Autodesk Inventor part; units mm, degrees
ref_plane "YZ Plane" through (0, 0, 0) normal (1, 0, 0) x (0, 1, 0)
ref_plane "XZ Plane" through (0, 0, 0) normal (0, 1, 0) x (-1, 0, 0)
ref_plane "XY Plane" through (0, 0, 0) normal (0, 0, 1) x (1, 0, 0)
sketch "Boceto1" plane through (0, 0, 0) normal (0, 1, 0) x (-1, 0, 0)
  line L0 (-5, 0) -> (-75.1, 0)
  line L1 (-80.1, -5) -> (-80.1, -91.5)
  line L2 (-75.1, -96.5) -> (-5, -96.5)
  line L3 (0, -91.5) -> (0, -5)
  arc A0 (0, -5) -> (-5, 0) centre (-5, -5) ccw
  arc A1 (-75.1, 0) -> (-80.1, -5) centre (-75.1, -5) ccw
  arc A2 (-80.1, -91.5) -> (-75.1, -96.5) centre (-75.1, -91.5) ccw
  arc A3 (-5, -96.5) -> (0, -91.5) centre (-5, -91.5) ccw
  point P0 (0, 0)
  point P1 (-80.1, -96.5)
  point P2 (-80.1, 0)
  point P3 (0, -96.5)
  dimension "d0" = 96.5
  dimension "d1" = 80.1
  dimension "d2" = 5
extrude "Extrusión1" add sketch "Boceto1" along normal blind 6
sketch "Boceto2" plane through (0, 0, 0) normal (0, -1, 0) x (1, 0, 0)
  circle A0 centre (10.2, -10.54) radius 2.5
  circle A1 centre (10.2, -16.54) radius 2.5
  circle A2 centre (7.06, -57.64) radius 2.4
  circle A3 centre (7.06, -62.64) radius 2.4
  circle A4 centre (7.06, -67.64) radius 2.4
  circle A5 centre (7.08, -75.21) radius 2.4
  circle A6 centre (7.08, -80.21) radius 2.4
  circle A7 centre (7.08, -85.21) radius 2.4
  point P0 (0, 0)
extrude "Extrusión2" cut sketch "Boceto2" against normal blind 10
sketch "Boceto3" plane through (0, 6, 0) normal (0, 1, 0) x (1, 0, 0)
  line L0 (6.9461, 7.6948) -> (13.2683, 7.6948)
  line L1 (13.2683, 7.6948) -> (13.2683, 19.5905)
  line L2 (13.2683, 19.5905) -> (6.9461, 19.5905)
  line L3 (6.9461, 19.5905) -> (6.9461, 7.6948)
  circle A0 centre (10.2, 16.54) radius 2.5
  circle A1 centre (10.2, 10.54) radius 2.5
  point P0 (0, 0)
extrude "Extrusión3" add sketch "Boceto3" along normal blind 15
fillet "Empalme1" radius 3 4 edges at (6.9461, 13.5, -19.5905) (6.9461, 13.5, -7.6948) (13.2683, 13.5, -7.6948) (13.2683, 13.5, -19.5905)
sketch "Boceto4" plane through (0, 6, 0) normal (0, 1, 0) x (1, 0, 0)
  line L0 (3.9852, 54.3304) -> (10.0586, 54.3304)
  line L1 (10.0586, 54.3304) -> (10.0586, 88.8384)
  line L2 (10.0586, 88.8384) -> (3.9852, 88.8384)
  line L3 (3.9852, 88.8384) -> (3.9852, 54.3304)
  circle A0 centre (7.06, 57.64) radius 2.4
  circle A1 centre (7.06, 62.64) radius 2.4
  circle A2 centre (7.06, 67.64) radius 2.4
  circle A3 centre (7.08, 75.21) radius 2.4
  circle A4 centre (7.08, 80.21) radius 2.4
  circle A5 centre (7.08, 85.21) radius 2.4
  point P0 (0, 0)
extrude "Extrusión4" add sketch "Boceto4" along normal blind 15
fillet "Empalme2" radius 3 4 edges at (3.9852, 13.5, -54.3304) (3.9852, 13.5, -88.8384) (10.0586, 13.5, -88.8384) (10.0586, 13.5, -54.3304)
properties part number "Tapa Case"
The listing builds one solid part. Answer for the finished solid, in the listing's coordinates (mm). A direction names the side the tool comes from. Give positions to 0.01 mm unless a question says otherwise; leave off trailing zeros. Loops run counter-clockwise (first coordinate to the right, second up) from the corner with the lowest first, then second, coordinate; pieces in that order, holes last. Notation, with made-up numbers: (12, 10.25) - (37, 10.25) arc R9 ccw to (37, 27.25) - close; hole circle Ø7 at (-32, -37). An arc over 180 degrees is marked (long way). Return JSON: item names as keys, results as strings. Group by question number.
1. Given pin 1 Ø1.8 at (y, z) = (10.5, -14.5) entering from -X; pin 2 Ø5.5 at (x, z) = (7.06, -57.64) entering from -Y; pin 3 Ø6 at (x, z) = (37, -33) entering from +Y; pin 4 Ø4 at (y, z) = (12, -61) entering from +X, each flat-ended and moving along its own axis, determine where each tip first touches the part or whether it passes through.
2. Which of the six approach directions +Z, -Z, +X, -X, +Y, -Y give full straight-line access (tool end or side, diameter ignored) to faces 4 (the flat face through (10.059, 13, -71)), 5 (the cylindrical face through (9.16, 13.6, -55.19)), 6 (the cylindrical face through (4.887, 13.605, -87.983)), 7 (the cylindrical face through (7.8, 13.6, -8.6))?
3. Find section D-D (x = 37). Write down the section's boundary in (y, z).
4. Find section A-A (y = 18). State how many separate pieces and enclosed holes the cut face has, then the cut area to 3 significant figures.
5. Find section B-B (z = -80.21). Write down the section's boundary in (x, y), then the cut area to 3 significant figures.
6. Determine the mould class of faces 1 (the flat face through (0, 3, -49)), 2 (the flat face through (40, 3, 0)), 3 (the cylindrical face through (5.155, 10.353, -64.1)) for opening direction Z: pulls with the +Z half, pulls with the -Z half, needs draft (parallel to the pull), parting line crosses it, or undercut.
7. Straight lines are drawn through the part: line 1 (X direction, y = 11.5, z = -85.21); line 2 (Y direction, x = 48, z = -66); line 3 (Z direction, x = 11.5, y = 9.25). For each, find the intervals that lie inside material, in ascending order. Write a range as [from, to].
Verdict:
{
 "1": {"pin 1": "stops at x = 6.95", "pin 2": "stops at y = 0", "pin 3": "stops at y = 6", "pin 4": "stops at x = 10.06"},
 "2": {"face 4": "-Z, +X, +Y", "face 5": "+X, +Y", "face 6": "-Z, -X, +Y", "face 7": "+Z, -X, +Y"},
 "3": {"outline": "(0, -96.5) - (6, -96.5) - (6, 0) - (0, 0) - close"},
 "4": {"separate pieces": "2", "enclosed holes": "8", "area": "121 mm^2"},
 "5": {"outline": "(0, 0) - (4.68, 0) - (4.68, 21) - (3.99, 21) - (3.99, 6) - (0, 6) - close; (9.48, 0) - (80.1, 0) - (80.1, 6) - (10.06, 6) - (10.06, 21) - (9.48, 21) - close", "area": "471 mm^2"},
 "6": {"face 1": "needs draft", "face 2": "pulls with the +Z half", "face 3": "undercut"},
 "7": {"line 1": "x = [3.99, 4.68], [9.48, 10.06]", "line 2": "y = [0, 6]", "line 3": "z = [-19.33, -18.68], [-14.4, -12.68], [-8.4, -7.96]"}
}
